Build history of the part. All positions in model axes, mm. A direction names the side the tool comes from. Give positions to 0.01 mm unless a question says otherwise; leave off trailing zeros. Loops run counter-clockwise (first coordinate to the right, second up) from the corner with the lowest first, then second, coordinate; pieces in that order, holes last.
1) Flat gauge pins, fed straight in: P1, Ø5.5, axis at x = -24, y = 3, coming from the +Z side; P2, Ø8, axis at y = -7.5, z = -10, coming from the +X side; P3, Ø6.5, axis at x = 23, y = -1.5, coming from the +Z side; P4, Ø3, axis at x = -25.5, y = 4.8, coming from the +Z side. Where does each tip first touch, or does it go through?
2) Band-saw the part on C-C on x = 10.4. List the corners of the cut face in (y, z), then the cut area to 3 significant figures.
3) 3-axis set-ups, long thin cutter, end or side, ignore diameter. For faces 1 (the flat face through (24, 0, 2.5)), 2 (the flat face through (-20.4, 0, 5)), 3 (the flat face through (-24, 0, 0)), 4 (the flat face through (23, -2.9, -24)): which of +Z, -Z, +X, -X, +Y, -Y reach the whole face in a straight line?
4) Band-saw the part on A-A on x = 25.5. List the corners of the cut face in (y, z).
5) Band-saw the part on D-D on z = -9.5. List the corners of the cut face in (x, y), then the cut area to 3 significant figures.
6) Wall check: line 1 (Y direction, x = -25.5, z = 1.65); line 2 (X direction, y = 4.8, z = 0.8); line 3 (Z direction, x = -17, y = 1.75). Give the ranges that are in metal, low to high.
7) Two-plate mould, pull along Z, no slides. Class faces 5 (the flat face through (-20.4, 0, -13)), 6 (the flat face through (3, 0, -26)), 7 (the flat face through (24, 0, 0)): +Z half, -Z half, draft (parallel to the pull), parting line (faces both ways), or undercut.
8) Band-saw the part on B-B on y = -4.8. List the corners of the cut face in (x, z).
```python
from build123d import *

# Parameters (mm, degrees)
SKETCH1_W           = 54
SKETCH1_H           = 20
BOSS_EXTRUDE1_DEPTH = 2.5
SKETCH3_R           = 1.95
CUT_EXTRUDE1_DEPTH  = 2.5
SKETCH4_W           = 40.8
SKETCH4_H           = 20
BOSS_EXTRUDE2_DEPTH = 6
SKETCH5_W           = 40.8
SKETCH5_H           = 20
BOSS_EXTRUDE3_DEPTH = 26
SKETCH6_R           = 2.9
BOSS_EXTRUDE4_DEPTH = 3.5
SKETCH7_W           = 4
SKETCH7_H           = 5.8
BOSS_EXTRUDE5_DEPTH = 6


with BuildPart() as part:
    # Sketch1 → Boss-Extrude1 (new body)
    with BuildSketch(Plane.XY):
        Rectangle(SKETCH1_W, SKETCH1_H)
    extrude(amount=BOSS_EXTRUDE1_DEPTH)

    # Sketch3 → Cut-Extrude1 (cut)
    with BuildSketch(Plane.XY.offset(2.5)):
        with Locations((-25.5, 4.8)):
            Circle(SKETCH3_R)
        with Locations((-25.5, -4.8)):
            Circle(SKETCH3_R)
        with Locations((25.5, -4.8)):
            Circle(SKETCH3_R)
        with Locations((25.5, 4.8)):
            Circle(SKETCH3_R)
    extrude(amount=-CUT_EXTRUDE1_DEPTH, mode=Mode.SUBTRACT)

    # Sketch4 → Boss-Extrude2 (add)
    with BuildSketch(Plane.XY.offset(2.5)):
        Rectangle(SKETCH4_W, SKETCH4_H)
    extrude(amount=BOSS_EXTRUDE2_DEPTH)

    # Sketch5 → Boss-Extrude3 (add)
    with BuildSketch(Plane(origin=(0, 0, 0), x_dir=(-1, 0, 0), z_dir=(0, 0, -1))):
        Rectangle(SKETCH5_W, SKETCH5_H)
    extrude(amount=BOSS_EXTRUDE3_DEPTH)

    # Sketch6 → Boss-Extrude4 (add)
    with BuildSketch(Plane.XY.offset(8.5)):
        with Locations((10.4, 0)):
            Circle(SKETCH6_R)
    extrude(amount=BOSS_EXTRUDE4_DEPTH)

    # Sketch7 → Boss-Extrude5 (add)
    with BuildSketch(Plane(origin=(20.4, 0, 0), x_dir=(0, 0, -1), z_dir=(1, 0, 0))):
        with Locations((24, 0)):
            Rectangle(SKETCH7_W, SKETCH7_H)
    extrude(amount=BOSS_EXTRUDE5_DEPTH)


solid = part.part
```
Findings below:
1. P1: stops at z = 2.5
1. P2: stops at x = 20.4
1. P3: stops at z = 8.5
1. P4: passes through
2. outline: (-10, -26) - (10, -26) - (10, 8.5) - (2.9, 8.5) - (2.9, 12) - (-2.9, 12) - (-2.9, 8.5) - (-10, 8.5) - close
2. area: 710 mm2
3. face 1: +Z, +X, +Y, -Y
3. face 2: +Z, -X, +Y, -Y
3. face 3: -Z, -X, +Y, -Y
3. face 4: -Z, +X, -Y
4. outline: (-10, 0) - (-6.75, 0) - (-6.75, 2.5) - (-10, 2.5) - close; (-2.9, -26) - (2.9, -26) - (2.9, -22) - (-2.9, -22) - close; (-2.85, 0) - (2.85, 0) - (2.85, 2.5) - (-2.85, 2.5) - close; (6.75, 0) - (10, 0) - (10, 2.5) - (6.75, 2.5) - close
5. outline: (-20.4, -10) - (20.4, -10) - (20.4, 10) - (-20.4, 10) - close
5. area: 816 mm2
6. line 1: y = -10 to -6.75, -2.85 to 2.85, 6.75 to 10
6. line 2: x = -23.55 to 23.55
6. line 3: z = -26 to 8.5
7. face 5: draft
7. face 6: -Z half
7. face 7: undercut
8. outline: (-23.55, 0) - (-20.4, 0) - (-20.4, -26) - (20.4, -26) - (20.4, 0) - (23.55, 0) - (23.55, 2.5) - (20.4, 2.5) - (20.4, 8.5) - (-20.4, 8.5) - (-20.4, 2.5) - (-23.55, 2.5) - close
